```python
from build123d import *

# Parameters (mm, degrees)
SKETCH1_R           = 97.5
BOSS_EXTRUDE1_DEPTH = 12
SKETCH2_R           = 20
CUT_EXTRUDE1_DEPTH  = 139.407008493
SKETCH3_R           = 10
CUT_EXTRUDE2_DEPTH  = 7.448022
CIRPATTERN1_START   = 4.551977781
CIRPATTERN1_DEPTH   = 7.448022219


# Read off the part's stored shape, not the designer's step: CirPattern1
with BuildPart() as part:
    # Sketch1 → Boss-Extrude1 (new body)
    with BuildSketch(Plane(origin=(0, 0, 0), x_dir=(1, 0, 0), z_dir=(0, 1, 0))):
        with Locations(Location((0, 0, 0), (0, 0, 270))):
            Circle(SKETCH1_R)
    extrude(amount=BOSS_EXTRUDE1_DEPTH)

    # Sketch2 → Cut-Extrude1 (cut, through all)
    with BuildSketch(Plane(origin=(0, 0, 0), x_dir=(1, 0, 0), z_dir=(0, 1, 0))):
        with Locations(Location((0, 0, 0), (0, 0, 270))):
            Circle(SKETCH2_R)
    extrude(amount=CUT_EXTRUDE1_DEPTH, mode=Mode.SUBTRACT)

    # Sketch3 → Cut-Extrude2 (cut)
    with BuildSketch(Plane(origin=(0, 12, 0), x_dir=(1, 0, 0), z_dir=(0, 1, 0))):
        with Locations((-29.72284232, 0)):
            Circle(SKETCH3_R)
    extrude(amount=-CUT_EXTRUDE2_DEPTH, mode=Mode.SUBTRACT)

    # CirPattern1 outline → CirPattern1 (cut)
    with BuildSketch(Plane(origin=(0, 0, 0), x_dir=(1, 0, 0), z_dir=(0, 1, 0)).offset(CIRPATTERN1_START)):
        with BuildLine():
            ThreePointArc((8.295012814, 18.198702218), (10, 17.320508076), (11.613032029, 16.283042931))
            ThreePointArc((11.613032029, 16.283042931), (19.86142116, 34.400990559), (8.295012814, 18.198702218))
        make_face()
        with BuildLine():
            ThreePointArc((11.613032029, -16.283042931), (10, -17.320508076), (8.295012814, -18.198702218))
            ThreePointArc((8.295012814, -18.198702218), (19.86142116, -34.400990559), (11.613032029, -16.283042931))
        make_face()
    extrude(amount=CIRPATTERN1_DEPTH, mode=Mode.SUBTRACT)


solid = part.part
```
For this review, take the finished solid that the model builds, in its own axes (mm). A direction names the side the tool comes from. Round coordinates to 2 decimals unless told otherwise and drop trailing zeros. Write each loop counter-clockwise with the first axis right and the second up, starting at its lowest first coordinate (ties: lowest second). Pieces come first, ordered by that corner, then holes. Notation, with made-up numbers: (-21, 19) -> (0, 19) arc R7 ccw to (0, 29) -> close; hole circle Ø2 at (23.25, 10.25). An arc over 180 degrees is marked (long way). One line per question, with ' | ' between items. Start each with the question number.
1) Add section D-D (x = -48). Write out the cut boundary in (y, z), and give its area (3 significant figures).
2) Machinability: for faces 4 (the flat face through (15, 4.552, 26)), 5 (the flat face through (1.4, 12, 20.3)), which of the approach directions +Z, -Z, +X, -X, +Y, -Y give a long, thin tool a straight path to every point of the face, cutting with its end or side? Answer none if there is none.
3) For pin 1 Ø1 at (x, y) = (45.5, 7) entering from +Z; pin 2 Ø2 at (y, z) = (2.5, -63) entering from +X; pin 3 Ø22 at (x, z) = (-30, -0.5) entering from +Y; pin 4 Ø2 at (y, z) = (8, 77) entering from -X, all flat-tipped, find the tip position at first contact; note any pin that passes through.
4) Add section A-A (x = 0). Write out the cut boundary in (y, z).
5) Mouldability with a two-part tool opening along Z and no side actions: class faces 1 (the cylindrical face through (-86.5, 5.92, 44.99)), 2 (the cylindrical face through (-19.524, 5.916, -4.336)), 3 (the flat face through (-20.3, 0, -1.4)) as +Z half, -Z half, draft (parallel to the pull), parting line (faces both ways), or undercut.
6) Add section C-C (y = 9). Write out the cut boundary in (x, z).
7) Wall thickness on line 1 along X through (y, z) = (3.5, 0); line 2 along Z through (x, y) = (23, 8.75); line 3 along X through (y, z) = (10.5, -9): over which ranges is each line inside the solid? List them lowest first.
8) Add section B-B (z = 5.5). Write out the cut boundary in (x, y).
Reported:
1) outline: (0, -84.87) -> (12, -84.87) -> (12, 84.87) -> (0, 84.87) -> close | area: 2,040 mm²
2) face 4: +Y | face 5: +Z, -Z, +X, -X, +Y
3) pin 1: stops at z = 86.49 | pin 2: stops at x = 75.25 | pin 3: stops at y = 12 | pin 4: stops at x = -61.08
4) outline: (0, -97.5) -> (12, -97.5) -> (12, -20) -> (0, -20) -> close; (0, 20) -> (12, 20) -> (12, 97.5) -> (0, 97.5) -> close
5) face 1: parting line | face 2: undercut | face 3: draft
6) outline: circle Ø195 at (0, 0); hole (-19.91, -1.92) arc R20 ccw to (8.3, -18.2) arc R10 ccw (long way) to (11.61, -16.28) arc R20 ccw to (11.61, 16.28) arc R10 ccw (long way) to (8.3, 18.2) arc R20 ccw to (-19.91, 1.92) arc R10 ccw (long way) to start
7) line 1: x = -97.5 to -20, 20 to 97.5 | line 2: z = -94.75 to -31.55, -19.93 to 19.93, 31.55 to 94.75 | line 3: x = -97.08 to -34.08, -25.36 to -17.86, 17.86 to 97.08
8) outline: (-97.34, 0) -> (-19.23, 0) -> (-19.23, 12) -> (-21.37, 12) -> (-21.37, 4.55) -> (-38.07, 4.55) -> (-38.07, 12) -> (-97.34, 12) -> close; (19.23, 0) -> (97.34, 0) -> (97.34, 12) -> (19.23, 12) -> close
